```python
from build123d import *

# Parameters (mm, degrees)
SKETCH1_W           = 25.4
SKETCH1_H           = 25.4
SKETCH1_W_2         = 22.225
SKETCH1_H_2         = 22.225
BOSS_EXTRUDE1_DEPTH = 812.8
SKETCH2_R           = 3.2639
CUT_EXTRUDE1_DEPTH  = 814.593362805
SKETCH3_R           = 3.2639
SKETCH3_R_2         = 4.953
CUT_EXTRUDE2_DEPTH  = 814.593362805


with BuildPart() as part:
    # Sketch1 → Boss-Extrude1 (new body)
    with BuildSketch(Plane.XY):
        with Locations((12.7, 12.7)):
            Rectangle(SKETCH1_W, SKETCH1_H)
        with Locations((12.7, 12.7)):
            Rectangle(SKETCH1_W_2, SKETCH1_H_2, mode=Mode.SUBTRACT)
    extrude(amount=BOSS_EXTRUDE1_DEPTH)

    # Sketch2 → Cut-Extrude1 (cut, through all)
    with BuildSketch(Plane(origin=(25.4, 0, 0), x_dir=(0, 0, -1), z_dir=(1, 0, 0))):
        with Locations((-12.7, 12.7)):
            Circle(SKETCH2_R)
        with Locations((-38.1, 12.7)):
            Circle(SKETCH2_R)
        with Locations(Location((-774.7, 12.7, 0), (0, 0, 180))):
            Circle(SKETCH2_R)
        with Locations(Location((-800.1, 12.7, 0), (0, 0, 180))):
            Circle(SKETCH2_R)
    extrude(amount=-CUT_EXTRUDE1_DEPTH, mode=Mode.SUBTRACT)

    # Sketch3 → Cut-Extrude2 (cut, through all)
    with BuildSketch(Plane(origin=(25.4, 0, 0), x_dir=(0, 0, -1), z_dir=(1, 0, 0))):
        with Locations((-63.5, 12.7)):
            Circle(SKETCH3_R)
        with Locations((-736.6, 12.7)):
            Circle(SKETCH3_R)
        with Locations((-711.2, 12.7)):
            Circle(SKETCH3_R)
        with Locations((-685.8, 12.7)):
            Circle(SKETCH3_R)
        with Locations((-660.4, 12.7)):
            Circle(SKETCH3_R)
        with Locations((-635, 12.7)):
            Circle(SKETCH3_R)
        with Locations((-609.6, 12.7)):
            Circle(SKETCH3_R)
        with Locations((-495.3, 9.271)):
            Circle(SKETCH3_R_2)
        with Locations((-88.9, 12.7)):
            Circle(SKETCH3_R)
        with Locations((-114.3, 12.7)):
            Circle(SKETCH3_R)
        with Locations((-139.7, 12.7)):
            Circle(SKETCH3_R)
        with Locations((-165.1, 12.7)):
            Circle(SKETCH3_R)
        with Locations((-190.5, 12.7)):
            Circle(SKETCH3_R)
        with Locations((-215.9, 12.7)):
            Circle(SKETCH3_R)
        with Locations((-241.3, 12.7)):
            Circle(SKETCH3_R)
        with Locations((-266.7, 12.7)):
            Circle(SKETCH3_R)
        with Locations((-292.1, 12.7)):
            Circle(SKETCH3_R)
        with Locations((-317.5, 12.7)):
            Circle(SKETCH3_R)
        with Locations((-342.9, 12.7)):
            Circle(SKETCH3_R)
        with Locations((-368.3, 12.7)):
            Circle(SKETCH3_R)
        with Locations((-393.7, 12.7)):
            Circle(SKETCH3_R)
    extrude(amount=-CUT_EXTRUDE2_DEPTH, mode=Mode.SUBTRACT)


solid = part.part
```
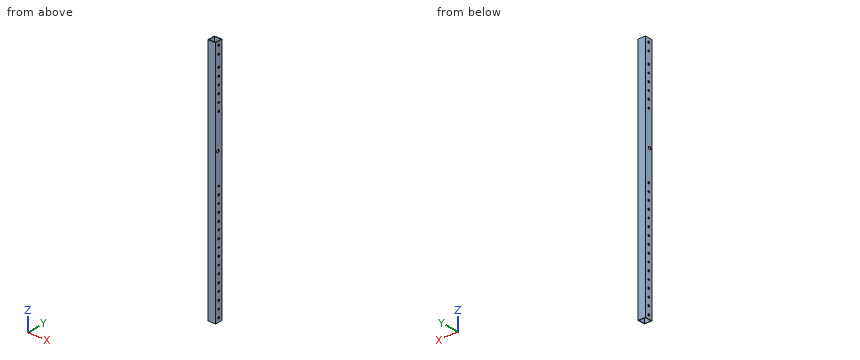
Part model, mm, in its own coordinate system. Round coordinates to 2 decimals unless told otherwise and drop trailing zeros. Loops run counter-clockwise (first coordinate to the right, second up) from the corner with the lowest first, then second, coordinate; pieces in that order, holes last. Notation, with made-up numbers: (-22, 5) -> (26, 5) arc R25 ccw to (26, 33) -> close; hole circle Ø9 at (15.5, -25). An arc over 180 degrees is marked (long way). Use CSV: the item, a comma, the result in double quotes. Start each with the question number.
1) Cut at A-A, the plane x = 13.25. Write the cut outline in (y, z), plus the area to 3 significant figures.
2) Wall check: L1, parallel to X at y = 13.25, z = 300; L2, parallel to Y at x = 24.8, z = 12.7. Give the ranges that are in metal, low to high. Write a range as [from, to].
3) Cut at B-B, the plane z = 533.5. Write the cut outline in (x, y).
Determined:
1,outline,"(0, 0) -> (1.59, 0) -> (1.59, 812.8) -> (0, 812.8) -> close; (23.81, 0) -> (25.4, 0) -> (25.4, 812.8) -> (23.81, 812.8) -> close"
1,area,"2,580 mm2"
2,L1,"x = [0, 1.59], [23.81, 25.4]"
2,L2,"y = [0, 9.44], [15.96, 25.4]"
3,outline,"(0, 0) -> (25.4, 0) -> (25.4, 25.4) -> (0, 25.4) -> close; hole (1.59, 1.59) -> (23.81, 1.59) -> (23.81, 23.81) -> (1.59, 23.81) -> close"
